Read the model definition and answer for the solid it produces. Units are mm, in the model's axes. Face numbers are marked on the shaded views. A direction names the side the tool comes from. Coordinates: 2 decimals unless noted, no trailing zeros. Loops run counter-clockwise (first coordinate to the right, second up) from the corner with the lowest first, then second, coordinate; pieces in that order, holes last.
Q1. The mould has two halves that part along Y. Classify the marked faces 6, 7, 8 and 9: pulls with the +Y half, pulls with the -Y half, needs draft (parallel to the pull), parting line crosses it, or undercut.
Q2. Section D-D (y = -20) is taken. Give the vertices of the cut face in (x, z).
Q3. Section C-C (x = -17.5) is taken. Give the vertices of the cut face in (y, z), then the cut area to 3 significant figures.
Q4. Which of the six approach directions +Z, -Z, +X, -X, +Y, -Y give full straight-line access (tool end or side, diameter ignored) to the marked faces 1, 2, 3, 4 and 5?
Q5. Straight lines are drawn through the part: line 1 (Y direction, x = -13, z = 0.2); line 2 (X direction, y = -28, z = 0.2); line 3 (X direction, y = -4, z = 2.45). For each, find the intervals that lie inside material, in ascending order.
Q6. Section A-A (z = -1.05) is taken. Give the vertices of the cut face in (x, y), then the cut area to 3 significant figures.
Q7. Flat-ended cylindrical pins translate along their axes: P1, Ø1.5, axis at y = -18.5, z = 1.5, coming from the -X side; P2, Ø0.5, axis at y = -25, z = 0.5, coming from the +X side; P3, Ø18.5, axis at x = -2.5, y = 2, coming from the +Z side. Find the tip coordinate at first contact, or state that the pin passes through.
Q8. Section B-B (y = 1.5) is taken. Give the vertices of the cut face in (x, z), then the cut area to 3 significant figures.
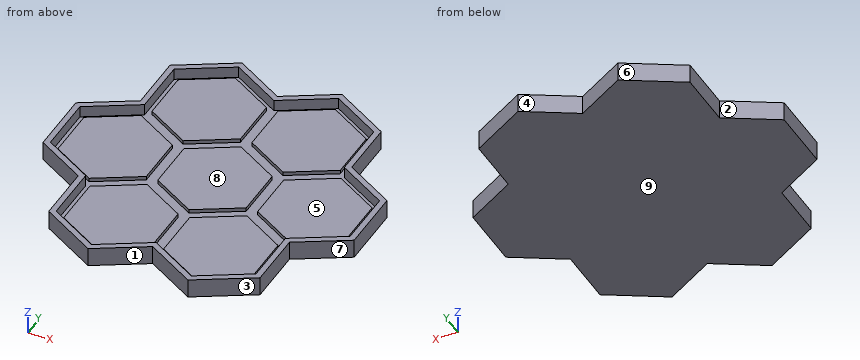
from build123d import *

# Parameters (mm, degrees)
F1_DEPTH = 2
F2_DEPTH = 1
F3_DEPTH = 3


with BuildPart() as f1:
    # F0 (on Top) → F1 (new body)
    with BuildSketch(Plane.XY):
        Polygon((-40.5, -8.371579), (-27.5, -15.877132), (-27.5, -30.888239), (-13, -39.259818), (0, -31.754265), (13, -39.259818), (27.5, -30.888239), (27.5, -15.877132), (40.5, -8.371579), (40.5, 8.371579), (27.5, 15.877132), (27.5, 30.888239), (13, 39.259818), (0, 31.754265), (-13, 39.259818), (-27.5, 30.888239), (-27.5, 15.877132), (-40.5, 8.371579), align=None)
        Polygon((-39, -7.505553), (-39, 7.505553), (-26, 15.011107), (-26, 30.022214), (-13, 37.527767), (0, 30.022214), (13, 37.527767), (26, 30.022214), (26, 15.011107), (39, 7.505553), (39, -7.505553), (26, -15.011107), (26, -30.022214), (13, -37.527767), (0, -30.022214), (-13, -37.527767), (-26, -30.022214), (-26, -15.011107), align=None, mode=Mode.SUBTRACT)
        Polygon((-26, 15.011107), (-39, 7.505553), (-39, -7.505553), (-26, -15.011107), (-26, -30.022214), (-13, -37.527767), (0, -30.022214), (13, -37.527767), (26, -30.022214), (26, -15.011107), (39, -7.505553), (39, 7.505553), (26, 15.011107), (26, 30.022214), (13, 37.527767), (0, 30.022214), (-13, 37.527767), (-26, 30.022214), align=None)
        Polygon((-13, -35.795717), (-24.5, -29.156189), (-24.5, -15.877132), (-13, -9.237604), (-1.5, -15.877132), (-1.5, -29.156189), align=None, mode=Mode.SUBTRACT)
        Polygon((-26, -13.279056), (-37.5, -6.639528), (-37.5, 6.639528), (-26, 13.279056), (-14.5, 6.639528), (-14.5, -6.639528), align=None, mode=Mode.SUBTRACT)
        Polygon((13, -9.237604), (24.5, -15.877132), (24.5, -29.156189), (13, -35.795717), (1.5, -29.156189), (1.5, -15.877132), align=None, mode=Mode.SUBTRACT)
        Polygon((0, 13.279056), (11.5, 6.639528), (11.5, -6.639528), (0, -13.279056), (-11.5, -6.639528), (-11.5, 6.639528), align=None, mode=Mode.SUBTRACT)
        Polygon((26, 13.279056), (37.5, 6.639528), (37.5, -6.639528), (26, -13.279056), (14.5, -6.639528), (14.5, 6.639528), align=None, mode=Mode.SUBTRACT)
        Polygon((-13, 35.795717), (-1.5, 29.156189), (-1.5, 15.877132), (-13, 9.237604), (-24.5, 15.877132), (-24.5, 29.156189), align=None, mode=Mode.SUBTRACT)
        Polygon((13, 35.795717), (24.5, 29.156189), (24.5, 15.877132), (13, 9.237604), (1.5, 15.877132), (1.5, 29.156189), align=None, mode=Mode.SUBTRACT)
        Polygon((-37.5, 6.639528), (-37.5, -6.639528), (-26, -13.279056), (-14.5, -6.639528), (-14.5, 6.639528), (-26, 13.279056), align=None)
        Polygon((-1.5, 15.877132), (-1.5, 29.156189), (-13, 35.795717), (-24.5, 29.156189), (-24.5, 15.877132), (-13, 9.237604), align=None)
        Polygon((24.5, 15.877132), (24.5, 29.156189), (13, 35.795717), (1.5, 29.156189), (1.5, 15.877132), (13, 9.237604), align=None)
        Polygon((24.5, -29.156189), (24.5, -15.877132), (13, -9.237604), (1.5, -15.877132), (1.5, -29.156189), (13, -35.795717), align=None)
        Polygon((-24.5, -15.877132), (-24.5, -29.156189), (-13, -35.795717), (-1.5, -29.156189), (-1.5, -15.877132), (-13, -9.237604), align=None)
        Polygon((11.5, -6.639528), (11.5, 6.639528), (0, 13.279056), (-11.5, 6.639528), (-11.5, -6.639528), (0, -13.279056), align=None)
        Polygon((37.5, -6.639528), (37.5, 6.639528), (26, 13.279056), (14.5, 6.639528), (14.5, -6.639528), (26, -13.279056), align=None)
    extrude(amount=-F1_DEPTH)

    # F0 (on Top) → F2 (join)
    with BuildSketch(Plane.XY):
        Polygon((-37.5, 6.639528), (-37.5, -6.639528), (-26, -13.279056), (-14.5, -6.639528), (-14.5, 6.639528), (-26, 13.279056), align=None)
        Polygon((-1.5, 15.877132), (-1.5, 29.156189), (-13, 35.795717), (-24.5, 29.156189), (-24.5, 15.877132), (-13, 9.237604), align=None)
        Polygon((24.5, 15.877132), (24.5, 29.156189), (13, 35.795717), (1.5, 29.156189), (1.5, 15.877132), (13, 9.237604), align=None)
        Polygon((37.5, -6.639528), (37.5, 6.639528), (26, 13.279056), (14.5, 6.639528), (14.5, -6.639528), (26, -13.279056), align=None)
        Polygon((24.5, -29.156189), (24.5, -15.877132), (13, -9.237604), (1.5, -15.877132), (1.5, -29.156189), (13, -35.795717), align=None)
        Polygon((-24.5, -15.877132), (-24.5, -29.156189), (-13, -35.795717), (-1.5, -29.156189), (-1.5, -15.877132), (-13, -9.237604), align=None)
        Polygon((11.5, -6.639528), (11.5, 6.639528), (0, 13.279056), (-11.5, 6.639528), (-11.5, -6.639528), (0, -13.279056), align=None)
    extrude(amount=F2_DEPTH)

    # F0 (on Top) → F3 (join)
    with BuildSketch(Plane.XY):
        Polygon((-40.5, -8.371579), (-27.5, -15.877132), (-27.5, -30.888239), (-13, -39.259818), (0, -31.754265), (13, -39.259818), (27.5, -30.888239), (27.5, -15.877132), (40.5, -8.371579), (40.5, 8.371579), (27.5, 15.877132), (27.5, 30.888239), (13, 39.259818), (0, 31.754265), (-13, 39.259818), (-27.5, 30.888239), (-27.5, 15.877132), (-40.5, 8.371579), align=None)
        Polygon((-39, -7.505553), (-39, 7.505553), (-26, 15.011107), (-26, 30.022214), (-13, 37.527767), (0, 30.022214), (13, 37.527767), (26, 30.022214), (26, 15.011107), (39, 7.505553), (39, -7.505553), (26, -15.011107), (26, -30.022214), (13, -37.527767), (0, -30.022214), (-13, -37.527767), (-26, -30.022214), (-26, -15.011107), align=None, mode=Mode.SUBTRACT)
    extrude(amount=F3_DEPTH)


solid = f1.part
Numbers:
1. face 6: pulls with the +Y half
1. face 7: pulls with the -Y half
1. face 8: undercut
1. face 9: needs draft
2. outline: (-27.5, -2) - (27.5, -2) - (27.5, 3) - (26, 3) - (26, 0) - (24.5, 0) - (24.5, 1) - (1.5, 1) - (1.5, 0) - (-1.5, 0) - (-1.5, 1) - (-24.5, 1) - (-24.5, 0) - (-26, 0) - (-26, 3) - (-27.5, 3) - close
3. outline: (-36.66, -2) - (36.66, -2) - (36.66, 3) - (34.93, 3) - (34.93, 0) - (33.2, 0) - (33.2, 1) - (11.84, 1) - (11.84, 0) - (8.37, 0) - (8.37, 1) - (-8.37, 1) - (-8.37, 0) - (-11.84, 0) - (-11.84, 1) - (-33.2, 1) - (-33.2, 0) - (-34.93, 0) - (-34.93, 3) - (-36.66, 3) - close
3. area: 217 mm2
4. face 1: +Z, -Z, -Y
4. face 2: +Z, -Z, -X, +Y
4. face 3: +Z, -Z, +X, -Y
4. face 4: +Z, -Z, +Y
4. face 5: +Z
5. line 1: y = -39.26 to -37.53, -35.8 to -9.24, 9.24 to 35.8, 37.53 to 39.26
5. line 2: x = -27.5 to -26, -24.5 to -1.5, 1.5 to 24.5, 26 to 27.5
5. line 3: x = -40.5 to -39, 39 to 40.5
6. outline: (-40.5, -8.37) - (-27.5, -15.88) - (-27.5, -30.89) - (-13, -39.26) - (0, -31.75) - (13, -39.26) - (27.5, -30.89) - (27.5, -15.88) - (40.5, -8.37) - (40.5, 8.37) - (27.5, 15.88) - (27.5, 30.89) - (13, 39.26) - (0, 31.75) - (-13, 39.26) - (-27.5, 30.89) - (-27.5, 15.88) - (-40.5, 8.37) - close
6. area: 4,510 mm2
7. P1: stops at x = -27.5
7. P2: stops at x = 27.5
7. P3: stops at z = 1
8. outline: (-40.5, -2) - (40.5, -2) - (40.5, 3) - (39, 3) - (39, 0) - (37.5, 0) - (37.5, 1) - (14.5, 1) - (14.5, 0) - (11.5, 0) - (11.5, 1) - (-11.5, 1) - (-11.5, 0) - (-14.5, 0) - (-14.5, 1) - (-37.5, 1) - (-37.5, 0) - (-39, 0) - (-39, 3) - (-40.5, 3) - close
8. area: 240 mm2
